For this review, use the dimensioned drawing (mm, ordinates from the lowest corner) and the shaded views. A direction names the side the tool comes from. Give positions to 0.01 mm unless a question says otherwise; leave off trailing zeros. Order: outer loops, then holes, each group sorted by start corner. A loop starts at its lowest first (then second) coordinate and runs counter-clockwise, first axis right, second up. Notation, with made-up numbers: M 66.25,81.25 L 118.25,81.25 A17 cw 118.25,95.25 Z; hole C 22.5,53 d5. An arc over 180 degrees is marked long. Use CSV: the item, a comma, the result in double quotes. Start each with the question number.
(1) Tool access review of the marked faces 1 and 2: name each direction out of +Z, -Z, +X, -X, +Y, -Y from which nothing blocks a thin tool from reaching the whole face with its end or side.
(2) Consider section B-B (y = 51). Write out the cut boundary in (x, z), and give its area (3 significant figures).
(3) Consider section C-C (x = 99.5). Write out the cut boundary in (y, z), and give its area (3 significant figures).
(4) Clearance check with flat-ended pins moving along their axes: P1, Ø8, axis at y = 44.5, z = 7, coming from the -X side; P2, Ø6, axis at x = 46, z = 6, coming from the -Y side; P3, Ø5, axis at y = 54.5, z = 4.5, coming from the +X side; P4, Ø7.5, axis at x = 113, z = 7, coming from the +Y side. State where each tip first meets the part, or that it passes through.
(5) Wall thickness on L1, parallel to X at y = 55.5, z = 7.5; L2, parallel to Y at x = 82, z = 7; L3, parallel to Y at x = 119, z = 4.25: over which ranges is each line inside the solid? List them lowest first. Write a range as from..to.
(6) Consider section A-A (z = 10.5). Write out the cut boundary in (x, y), and give its area (3 significant figures).
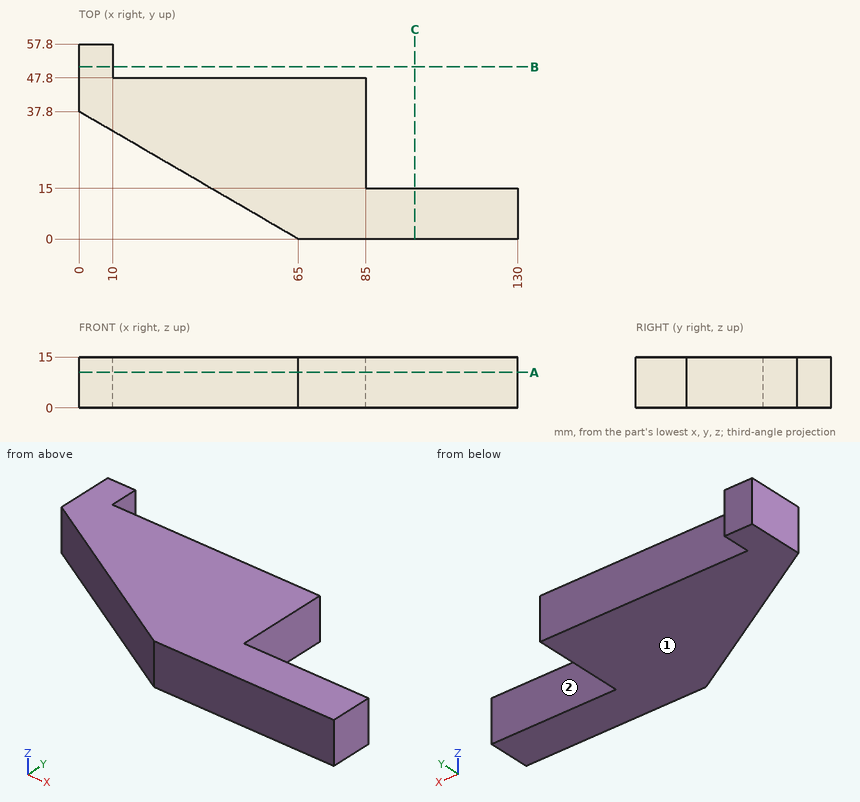
Check result:
1,face 1,"-Z, +X, -X, +Y, -Y"
1,face 2,"+Z, -Z, +X, +Y"
2,outline,"M 0,0 L 10,0 L 10,15 L 0,15 Z"
2,area,"150 mm^2"
3,outline,"M 0,0 L 15,0 L 15,15 L 0,15 Z"
3,area,"225 mm^2"
4,P1,"stops at x = 0"
4,P2,"stops at y = 9.3"
4,P3,"stops at x = 10"
4,P4,"stops at y = 15"
5,L1,"x = 0..10"
5,L2,"y = 0..47.8"
5,L3,"y = 0..15"
6,outline,"M 0,37.8 L 65,0 L 130,0 L 130,15 L 85,15 L 85,47.8 L 10,47.8 L 10,57.8 L 0,57.8 Z"
6,area,"3,610 mm^2"
